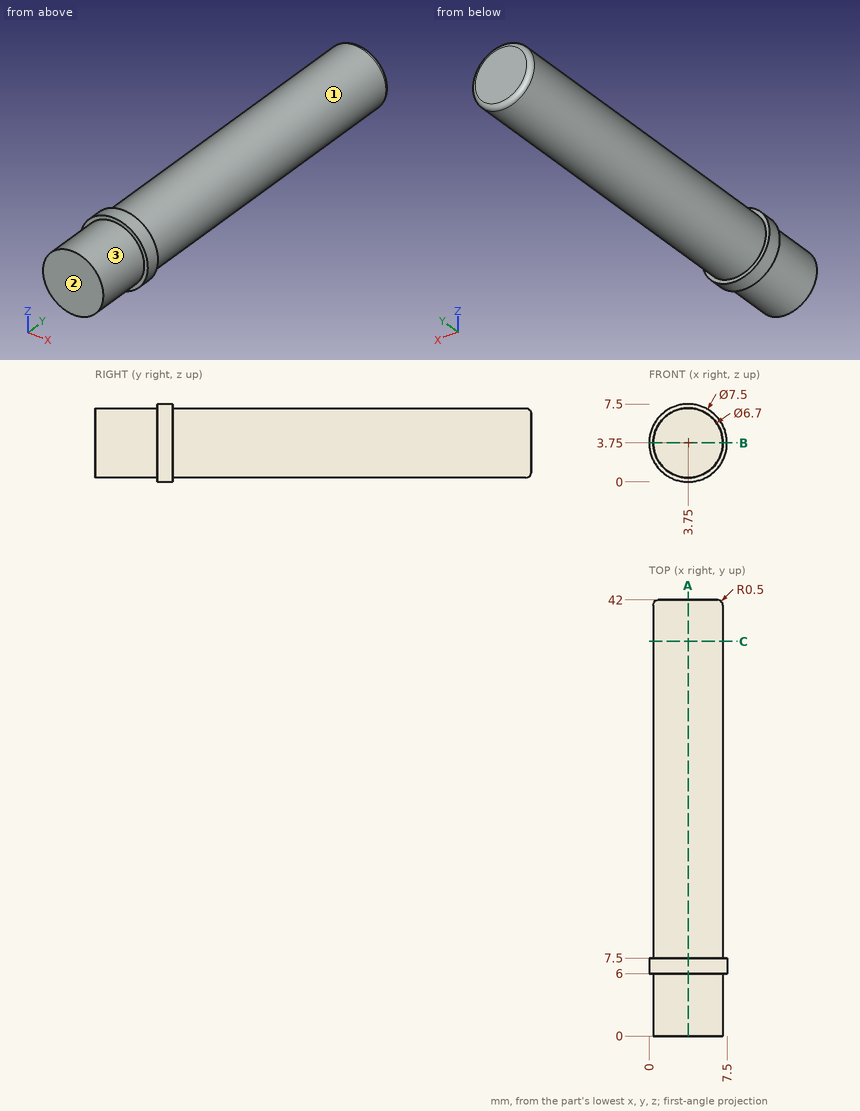
The figure shows three views and two pictorial views of one solid part (mm, origin at its lowest corner). Answer the questions. A direction names the side the tool comes from. Give positions to 0.01 mm unless a question says otherwise; leave off trailing zeros. Loops run counter-clockwise (first coordinate to the right, second up) from the corner with the lowest first, then second, coordinate; pieces in that order, holes last. Notation, with made-up numbers: (-30, 80.5) -> (12, 80.5) arc R22 cw to (12, 86.5) -> close; hole circle Ø1 at (15, -3). An arc over 180 degrees is marked (long way). Use CSV: the item, a comma, the result in double quotes.
1. The part is cut by section B-B (z = 3.75). Write down the section's boundary in (x, y), then the cut area to 3 significant figures.
Found:
outline,"(0, 6) -> (0.4, 6) -> (0.4, 0) -> (7.1, 0) -> (7.1, 6) -> (7.5, 6) -> (7.5, 7.5) -> (7.1, 7.5) -> (7.1, 41.5) arc R0.5 ccw to (6.6, 42) -> (0.9, 42) arc R0.5 ccw to (0.4, 41.5) -> (0.4, 7.5) -> (0, 7.5) -> close"
area,"282 mm^2"
2. The part is cut by section A-A (x = 3.75). Write down the section's boundary in (y, z), then the cut area to 3 significant figures.
Found:
outline,"(0, 0.4) -> (6, 0.4) -> (6, 0) -> (7.5, 0) -> (7.5, 0.4) -> (41.5, 0.4) arc R0.5 ccw to (42, 0.9) -> (42, 6.6) arc R0.5 ccw to (41.5, 7.1) -> (7.5, 7.1) -> (7.5, 7.5) -> (6, 7.5) -> (6, 7.1) -> (0, 7.1) -> close"
area,"282 mm^2"
3. A tool of negligible diameter and unlimited length cuts with its end or side. For the marked faces 1, 2 and 3, from which of +Z, -Z, +X, -X, +Y, -Y can it reach the whole face along a straight path? Write none if from no direction.
Found:
face 1,"+Y"
face 2,"+Z, -Z, +X, -X, -Y"
face 3,"-Y"
4. Flat-ended cylindrical pins translate along their axes: pin 1 Ø1 at (y, z) = (15.5, 6) entering from -X; pin 2 Ø1.5 at (x, y) = (1.5, 15.5) entering from -Z. Find the tip coordinate at first contact, or state that the pin passes through.
Found:
pin 1,"x = 0.89"
pin 2,"z = 0.75"
5. Straight lines are drawn through the part: line 1 (X direction, y = 19.5, z = 2); line 2 (X direction, y = 39, z = 3.75). For each, find the intervals that lie inside material, in ascending order.
Found:
line 1,"0.89 to 6.61"
line 2,"0.4 to 7.1"
6. The part is cut by section C-C (y = 38). Write down the section's boundary in (x, z), then the cut area to 3 significant figures.
Found:
outline,"circle Ø6.7 at (3.75, 3.75)"
area,"35.3 mm^2"
